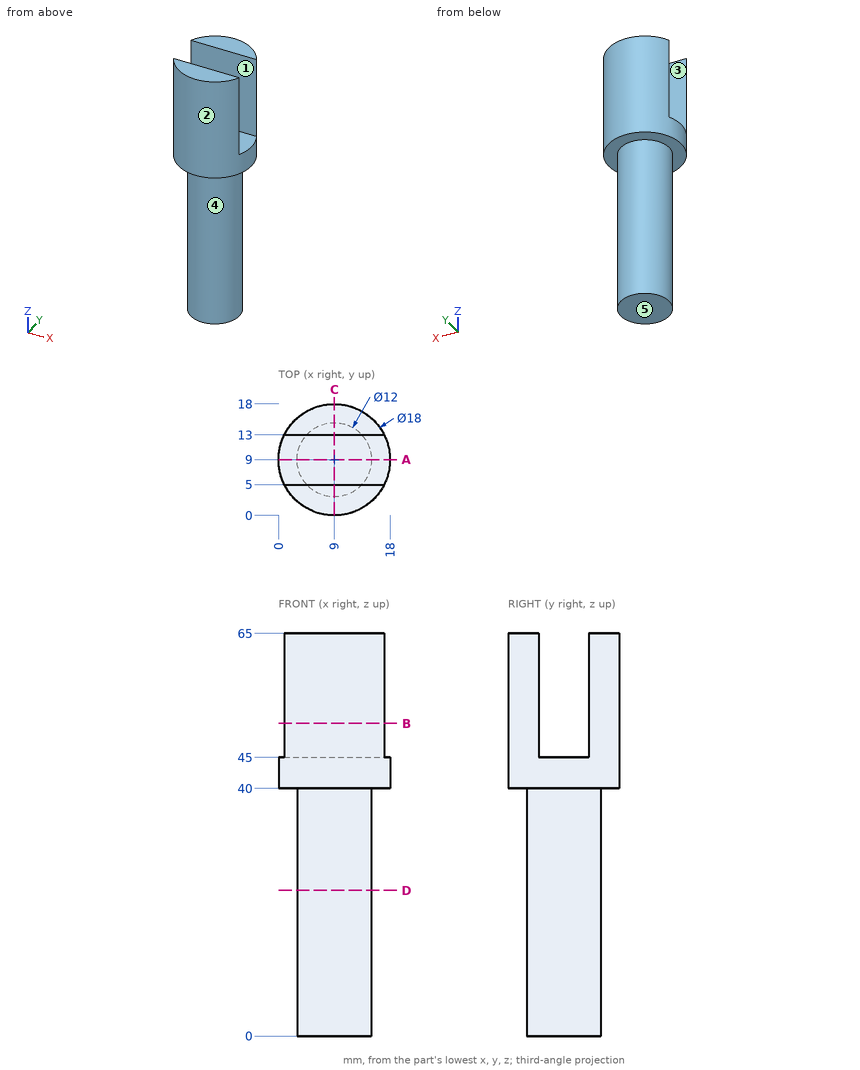
Job drawing, mm, ordinate dimensions from the low corner. One solid piece. A direction names the side the tool comes from. Round coordinates to 2 decimals unless told otherwise and drop trailing zeros. Loops run counter-clockwise (first coordinate to the right, second up) from the corner with the lowest first, then second, coordinate; pieces in that order, holes last.
(1) Cut at B-B (z = 50.5). Give the cut face in (x, y).
(2) Drop flat-ended pins along their axis: pin 1 (1.5 mm diameter, centred on x = 15, z = 54.5, fed in from -Y); pin 2 (3 mm diameter, centred on x = 4, z = 42.5, fed in from -Y); pin 3 (6 mm diameter, centred on y = 14, z = 9, fed in from -X). Give the stop position or say it passes through.
(3) Cut at D-D (z = 23.5). Give the cut face in (x, y).
(4) Two-plate mould, pull along Y, no slides. Class the marked faces 3, 4 and 5: +Y half, -Y half, draft (parallel to the pull), parting line (faces both ways), or undercut.
(5) Which spindle directions (+Z, -Z, +X, -X, +Y, -Y) get a long thin tool onto all of the face, cutting with end or side? Do the marked faces 1 and 2. Say none if no direction does.
(6) Cut at A-A (y = 9). Give the cut face in (x, z), plus the area to 3 significant figures.
(7) Cut at C-C (x = 9). Give the cut face in (y, z).
(8) Wall check: line 1 along Y through (x, z) = (9, 52); line 2 along Z through (x, y) = (10.5, 7.75); line 3 along Z through (x, y) = (1.5, 11.75). Give the ranges that are in metal, low to high.
Findings below:
1. outline: (0.94, 5) arc R9 ccw to (17.06, 5) - close; (0.94, 13) - (17.06, 13) arc R9 ccw to start
2. pin 1: stops at y = 1.69
2. pin 2: stops at y = 0.71
2. pin 3: stops at x = 3.34
3. outline: circle Ø12 at (9, 9)
4. face 3: undercut
4. face 4: parting line
4. face 5: draft
5. face 1: +Z, +X, -X
5. face 2: +Z, -Z
6. outline: (0, 40) - (3, 40) - (3, 0) - (15, 0) - (15, 40) - (18, 40) - (18, 45) - (0, 45) - close
6. area: 570 mm2
7. outline: (0, 40) - (3, 40) - (3, 0) - (15, 0) - (15, 40) - (18, 40) - (18, 65) - (13, 65) - (13, 45) - (5, 45) - (5, 65) - (0, 65) - close
8. line 1: y = 0 to 5, 13 to 18
8. line 2: z = 0 to 45
8. line 3: z = 40 to 45
